Could you check a few things on this model? Use its own coordinates, in mm. A direction names the side the tool comes from. Give positions to 0.01 mm unless a question says otherwise; leave off trailing zeros. Order: outer loops, then holes, each group sorted by start corner. A loop starts at its lowest first (then second) coordinate and runs counter-clockwise, first axis right, second up. Notation, with made-up numbers: (-7.75, 84) -> (31.25, 84) arc R20 cw to (31.25, 120) -> close; hole circle Ø3 at (13.25, 31.25). An arc over 180 degrees is marked (long way). One line per item, written item: value.
```python
from build123d import *
from build123d.topology import SkipClean

# Parameters (mm, degrees)
BOSS_EXTRUDE1_DEPTH   = 3.81
BODY_MOVE_COPY2_ANGLE = 180
BOSS_EXTRUDE2_START   = -25.4
SKETCH2_R             = 9.5
BOSS_EXTRUDE2_DEPTH   = 146.05
LPATTERN1_COUNT       = 3
LPATTERN1_PITCH       = 146.05
BODY_MOVE_COPY3_ANGLE = 120
BODY_MOVE_COPY4_ANGLE = 120
BOSS_EXTRUDE3_START   = 17.94
SKETCH3_R             = 9.5
BOSS_EXTRUDE3_DEPTH   = 17.94
SKETCH4_R             = 9.5
BOSS_EXTRUDE4_DEPTH   = 17.94


with BuildPart() as part:
    # Sketch1 → Boss-Extrude1 (new, symmetric)
    with BuildSketch(Plane(origin=(0, 0, 0), x_dir=(1, 0, 0), z_dir=(0, 1, 0))):
        with BuildLine():
            Line((-5.499261314, 15.875), (-10.998522628, 6.35))
            ThreePointArc((-10.998522628, 6.35), (0, -12.7), (10.998522628, 6.35))
            Line((10.998522628, 6.35), (5.499261314, 15.875))
            ThreePointArc((5.499261314, 15.875), (0, 19.05), (-5.499261314, 15.875))
        make_face()
    extrude(amount=BOSS_EXTRUDE1_DEPTH, both=True)


with BuildPart() as body_2:
    # Body-Move_Copy1: copy of part
    add(part.part.moved(Location((0, 60.96, 0))))


with BuildPart() as body_2_1:
    # Body-Move_Copy2: moved
    add(body_2.part.rotate(Axis((0, 0, 0), (0, 1, 0)), BODY_MOVE_COPY2_ANGLE))


with BuildPart() as part_1:
    add(part.part)

    add(body_2_1.part)  # Boss-Extrude2 merges body 2
    # Sketch2 → Boss-Extrude2 (add)
    with BuildSketch(Plane(origin=(0, 0, 0), x_dir=(1, 0, 0), z_dir=(0, 1, 0)).offset(BOSS_EXTRUDE2_START)):
        with Locations(Location((0, 0, 0), (0, 0, 270))):
            Circle(SKETCH2_R)
    extrude(amount=BOSS_EXTRUDE2_DEPTH)


with BuildPart() as lpattern1_1:
    # LPattern1: pattern copy
    add(part_1.part.moved(Location(Vector(0, 1, 0) * (1 * LPATTERN1_PITCH))))


with BuildPart() as lpattern1_2:
    # LPattern1: pattern copy
    add(part_1.part.moved(Location(Vector(0, 1, 0) * (2 * LPATTERN1_PITCH))))


with BuildPart() as lpattern1_1_1:
    # Body-Move_Copy3: moved
    add(lpattern1_1.part.rotate(Axis((0, 0, 0), (0, 1, 0)), BODY_MOVE_COPY3_ANGLE))


with BuildPart() as lpattern1_2_1:
    # Body-Move_Copy4: moved
    add(lpattern1_2.part.rotate(Axis((0, 0, 0), (0, -1, 0)), BODY_MOVE_COPY4_ANGLE))


with BuildPart() as part_2:
    with SkipClean():  # the faces are left unmerged after this step: merging them gives an invalid solid
        add(part_1.part)

        # Sketch3 → Boss-Extrude3 (add)
        with BuildSketch(Plane.XZ.offset(25.4).offset(BOSS_EXTRUDE3_START)):
            with Locations(Location((0, 0, 0), (0, 0, 210))):
                Circle(SKETCH3_R)
        extrude(amount=-BOSS_EXTRUDE3_DEPTH)

    # Combine1: union LPattern1_1, LPattern1_2
    add(lpattern1_1_1.part)
    add(lpattern1_2_1.part)

    # Sketch4 → Boss-Extrude4 (add)
    with SkipClean():  # the faces are left unmerged after this step: merging them gives an invalid solid
        with BuildSketch(Plane(origin=(0, 412.75, 0), x_dir=(1, 0, 0), z_dir=(0, 1, 0))):
            with Locations(Location((0, 0, 0), (0, 0, 270))):
                Circle(SKETCH4_R)
        extrude(amount=BOSS_EXTRUDE4_DEPTH)


solid = part_2.part
```
1) If I drill on line 1 along Y through (x, z) = (-12, 1); line 2 along Y through (x, z) = (6, -12); line 3 along Y through (x, z) = (-2.5, 17), over which ranges is the centre line in solid material (lowest first)?
Answer below:
line 1: y = -3.81 to 3.81, 57.15 to 64.77, 142.24 to 149.86, 203.2 to 210.82, 288.29 to 295.91, 349.25 to 356.87
line 2: y = -3.81 to 3.81, 203.2 to 210.82
line 3: y = 57.15 to 64.77
2) Suppose I cut it at A-A, the plane y = 230. Write out the boundary of the cut face in (x, z).
Answer below:
outline: circle Ø19 at (0, 0)
3) We'd pull the mould along Y, two halves only. Please class faces 5 (the cylindrical face through (0.09, 0.05, -19.05)), 6 (the flat face through (-9, 142.24, 4)), 7 (the flat face through (0, 430.69, 0)): +Y half, -Y half, draft (parallel to the pull), parting line (faces both ways), or undercut.
Answer below:
face 5: draft
face 6: undercut
face 7: +Y half
4) For faces 1 (the flat face through (-6, 146, 12.7)), 2 (the flat face through (-8.287, 61.013, 11.046)), 3 (the flat face through (13.8, 292.2, -1.5)), 4 (the cylindrical face through (-10.808, 292.153, -6.67)), which set-ups out of +Z, -Z, +X, -X, +Y, -Y let a thin tool reach every point of the face, with its end or its side?
Answer below:
face 1: +Z, +X, -X, +Y
face 2: +Z, -X, -Y
face 3: -Z, +X, +Y
face 4: none
5) For P1, Ø5, axis at x = 5, z = -13.5, coming from the +Y side; P2, Ø5, axis at x = 13.5, z = -8.5, coming from the +Y side; P3, Ø1.5, axis at x = 6.5, y = 303, coming from the -Z side, each with a flat end and sliding along its axis, tell me the tip position at first contact or that it passes through.
Answer below:
P1: stops at y = 356.87
P2: stops at y = 210.82
P3: stops at z = -7.56
